Autodesk Inventor part; units mm, degrees
ref_plane "YZ Plane" through (0, 0, 0) normal (1, 0, 0) x (0, 1, 0)
ref_plane "XZ Plane" through (0, 0, 0) normal (0, 1, 0) x (-1, 0, 0)
ref_plane "XY Plane" through (0, 0, 0) normal (0, 0, 1) x (1, 0, 0)
sketch "Эскиз1" plane through (0, 0, 0) normal (0, 1, 0) x (-1, 0, 0)
  line L0 (0, 0) -> (9, 0)
  line L1 (9, 0) -> (9, -2.4)
  line L2 (9, -22) -> (0, -22)
  line L3 (0, -22) -> (0, 0)
  line L4 (9, -22) -> (34.6, -22)
  line L5 (34.6, -22) -> (34.6, -19.6)
  line L6 (34.6, -19.6) -> (9, -19.6)
  line L7 (9, -11) -> (0, -11)
  line L8 (9, 0) -> (34.6, 0)
  line L9 (34.6, 0) -> (34.6, -2.4)
  line L10 (34.6, -2.4) -> (9, -2.4)
  line L11 (9, -2.4) -> (9, -22)
  line L12 (4.5, -6) -> (4.5, -16) construction
  line L13 (3, -6) -> (3, -16)
  line L14 (6, -16) -> (6, -6)
  arc A0 (6, -6) -> (3, -6) centre (4.5, -6) ccw
  arc A1 (3, -16) -> (6, -16) centre (4.5, -16) ccw
  point P0 (4.5, -11)
  dimension "d0" = 9
  dimension "d1" = 22
  dimension "d2" = 25.6
  dimension "d3" = 2.4
  dimension "d4" = 5
  dimension "d5" = 3
  dimension "d6" = 30.1
extrude "Выдавливание1" add sketch "Эскиз1" along normal blind 2.4 contours L0 L1 L11 L7 L14 A0 L13 L3 | L8 L9 L10 L1 | L7 L13 A1 L14 L11 L2 L3 | L11 L6 L5 L4
properties part number "FixScan"
For this review, take the finished solid that the model builds, in its own axes (mm). A direction names the side the tool comes from. Round coordinates to 2 decimals unless told otherwise and drop trailing zeros. Loops run counter-clockwise (first coordinate to the right, second up) from the corner with the lowest first, then second, coordinate; pieces in that order, holes last. Notation, with made-up numbers: (-7.5, 50) - (39.5, 50) arc R24 ccw to (39.5, 61) - close; hole circle Ø6 at (53.25, 19). An arc over 180 degrees is marked (long way). Use one line per item in the form item = value.
Item 1: Consider section A-A on x = -10. Write out the cut boundary in (y, z).
Answers:
outline = (0, -22) - (2.4, -22) - (2.4, -19.6) - (0, -19.6) - close; (0, -2.4) - (2.4, -2.4) - (2.4, 0) - (0, 0) - close
Item 2: Tool access review of faces 5 (the flat face through (-9, 1, -11)), 6 (the cylindrical face through (-4.5, 1.2, -4.5)), 7 (the flat face through (-8, 0, -12)): name each direction out of +Z, -Z, +X, -X, +Y, -Y from which nothing blocks a thin tool from reaching the whole face with its end or side.
Answers:
face_5 = -X, +Y, -Y
face_6 = +Y, -Y
face_7 = +Z, -Z, +X, -X, -Y
Item 3: Clearance check with flat-ended pins moving along their axes: P1, Ø0.7, axis at y = 1, z = -9, coming from the -X side; P2, Ø3, axis at x = -11, z = -9, coming from the +Y side. State where each tip first meets the part, or that it passes through.
Answers:
P1 = -9
P2 = through
Item 4: For line 1 (Z direction, x = -23.5, y = 0.9); line 2 (X direction, y = 2.15, z = -10.5); line 3 (X direction, y = 0.1, z = -17), list the stretches that pass through material, from the lowest coordinate up.
Answers:
line_1 = -22 to -19.6, -2.4 to 0
line_2 = -9 to -6, -3 to 0
line_3 = -9 to -5.62, -3.38 to 0
Item 5: Consider section C-C on y = 1.05. Write out the cut boundary in (x, z), then the cut area to 3 significant figures.
Answers:
outline = (-34.6, -22) - (0, -22) - (0, 0) - (-34.6, 0) - (-34.6, -2.4) - (-9, -2.4) - (-9, -19.6) - (-34.6, -19.6) - close; hole (-6, -16) arc R1.5 ccw to (-3, -16) - (-3, -6) arc R1.5 ccw to (-6, -6) - close
area = 284 mm^2
Item 6: Consider section B-B on z = -12.25. Write out the cut boundary in (x, y), then the cut area to 3 significant figures.
Answers:
outline = (-9, 0) - (-6, 0) - (-6, 2.4) - (-9, 2.4) - close; (-3, 0) - (0, 0) - (0, 2.4) - (-3, 2.4) - close
area = 14.4 mm^2
Item 7: Mouldability with a two-part tool opening along Z and no side actions: class faces 1 (the flat face through (-3, 1, -11)), 2 (the flat face through (-22, 1, -19.6)), 3 (the flat face through (-34.6, 1, -21)), 4 (the flat face through (-17, 1, 0)) as +Z half, -Z half, draft (parallel to the pull), parting line (faces both ways), or undercut.
Answers:
face_1 = undercut
face_2 = undercut
face_3 = draft
face_4 = +Z half
